from build123d import *

# Parameters (mm, degrees)
SKETCH_W     = 133
SKETCH_H     = 80
PAD_DEPTH    = 10
PAD001_DEPTH = 24


with BuildPart() as part:
    # Sketch → Pad (new body)
    with BuildSketch(Plane.XY):
        Rectangle(SKETCH_W, SKETCH_H)
    extrude(amount=PAD_DEPTH)

    # Sketch001 → Pad001 (join)
    with BuildSketch(Plane.XY):
        with BuildLine():
            Line((-66.5, -40), (-66.5, 40))
            Line((-66.5, 40), (-54, 40))
            Line((-54, 40), (-54, 38))
            Line((-54, 38), (-57, 38))
            Line((-57, 38), (-57, 32))
            Line((-57, 32), (-54, 32))
            Line((-54, 32), (-54, 30))
            Line((-54, 30), (-57, 30))
            Line((-57, 30), (-57, -32))
            Line((-57, -32), (-55.06066, -33.93934))
            ThreePointArc((-55.06066, -36.06066), (-54.62132, -35), (-55.06066, -33.93934))
            Line((-55.06066, -36.06066), (-57, -38))
            Line((-57, -38), (-57, -40))
            Line((-57, -40), (-66.5, -40))
        make_face()
    extrude(amount=PAD001_DEPTH)


solid = part.part
The model under review builds one solid part; all positions refer to its coordinate system, in mm. A direction names the side the tool comes from. Coordinates: 2 decimals unless noted, no trailing zeros. Write each loop counter-clockwise with the first axis right and the second up, starting at its lowest first coordinate (ties: lowest second). Pieces come first, ordered by that corner, then holes. Notation, with made-up numbers: M -22,-4 L -17,-4 A22 cw -17,6 Z; hole C -8.75,11 d11. An arc over 180 degrees is marked long. Put each result on its own line as item: value.
1) For faces 5 (the flat face through (-62, 1, 24)), 6 (the flat face through (-57, -1, 17)), list the 3-axis set-ups (+Z, -Z, +X, -X, +Y, -Y) from which the entire face can be reached by the end or side of a thin tool; tool diameter is ignored.
Computed:
face 5: +Z, +X, -X, +Y, -Y
face 6: +Z, +X
2) Add section A-A on z = 16.25. Give the boundary of the cut face in (x, y), then the cut area to 3 significant figures.
Computed:
outline: M -66.5,-40 L -57,-40 L -57,-38 L -55.06,-36.06 A1.5 ccw -55.06,-33.94 L -57,-32 L -57,30 L -54,30 L -54,32 L -57,32 L -57,38 L -54,38 L -54,40 L -66.5,40 Z
area: 781 mm2
3) Draft analysis for pull direction Y (two halves, no side actions). For faces 1 (the flat face through (66.5, -1, 5)), 2 (the flat face through (-55, 38, 17)), 3 (the flat face through (-1, 40, 6)), 4 (the flat face through (-1, -40, 6)), state which applies: released by +Y, released by -Y, zero draft, split by the parting line, or undercut.
Computed:
face 1: zero draft
face 2: undercut
face 3: released by +Y
face 4: released by -Y
4) Clearance check with flat-ended pins moving along their axes: pin 1 Ø0.6 at (y, z) = (-38.5, 18) entering from +X; pin 2 Ø1 at (x, y) = (-35.5, -26.5) entering from +Z; pin 3 Ø0.9 at (x, z) = (-56, 19) entering from -Y. State where each tip first meets the part, or that it passes through.
Computed:
pin 1: stops at x = -57
pin 2: stops at z = 10
pin 3: stops at y = -37.45
5) Wall thickness on probe 1 along Z at (x, y) = (13.5, 22); probe 2 along X at (y, z) = (5, 23.25): over which ranges is each line inside the solid? List them lowest first. Write a range as [from, to].
Computed:
probe 1: z = [0, 10]
probe 2: x = [-66.5, -57]
6) Add section B-B on y = -13. Give the boundary of the cut face in (x, z).
Computed:
outline: M -66.5,0 L 66.5,0 L 66.5,10 L -57,10 L -57,24 L -66.5,24 Z
7) Add section C-C on x = -52. Give the boundary of the cut face in (y, z).
Computed:
outline: M -40,0 L 40,0 L 40,10 L -40,10 Z
